Source: CAD feature listing. Evaluate the final solid. Frame: model axes, mm. A direction names the side the tool comes from. Give positions to 0.01 mm unless a question says otherwise; leave off trailing zeros. Loops run counter-clockwise (first coordinate to the right, second up) from the corner with the lowest first, then second, coordinate; pieces in that order, holes last.
```python
from build123d import *

# Parameters (mm, degrees)
EXTRUDE_1_DEPTH     = 1.5
SKETCH_3_R          = 0.9
EXTRUDE_2_DEPTH     = 2
SKETCH_4_R          = 0.9
EXTRUDE_3_DEPTH     = 2
SKETCH_5_R          = 1.1
EXTRUDE_4_DEPTH     = 2
FILLET_1_R          = 2
SKETCH_6_R          = 0.9
CUT_EXTRUDE_1_DEPTH = 10
SKETCH_7_R          = 1
CUT_EXTRUDE_2_DEPTH = 10
SKETCH_8_R          = 0.9
EXTRUDE_5_DEPTH     = 3
CUT_EXTRUDE_3_DEPTH = 3


with BuildPart() as part:
    # 草图1 → 凸台-拉伸1 (new body)
    with BuildSketch(Plane(origin=(0, 0, 0), x_dir=(1, 0, 0), z_dir=(0, 1, 0))):
        Polygon((15.5, 26.846787517), (-15.5, 26.846787517), (-31, 0), (-15.5, -26.846787517), (15.5, -26.846787517), (31, 0), align=None)
    extrude(amount=EXTRUDE_1_DEPTH)

    # 草图3 → 凸台-拉伸2 (add)
    with BuildSketch(Plane(origin=(16, 0, 0), x_dir=(0, 0, -1), z_dir=(1, 0, 0))):
        Polygon((-4, 1.5), (-2.5, 8.5), (2.5, 8.5), (4, 1.5), align=None)
        with Locations((0, 6)):
            Circle(SKETCH_3_R, mode=Mode.SUBTRACT)
    extrude_2 = extrude(amount=-EXTRUDE_2_DEPTH)

    # 草图4 → 凸台-拉伸3 (add)
    with BuildSketch(Plane(origin=(17.8, 0, 0), x_dir=(0, 0, -1), z_dir=(1, 0, 0))):
        Polygon((-4, 1.5), (4, 1.5), (2.5, 8.5), (-2.5, 8.5), align=None)
        with Locations((0, 6)):
            Circle(SKETCH_4_R, mode=Mode.SUBTRACT)
    extrude_3 = extrude(amount=EXTRUDE_3_DEPTH)

    # 镜向3: 凸台-拉伸2, 凸台-拉伸3 across plane
    add(extrude_2.mirror(Plane(origin=(0, 0, 0), x_dir=(0, 0, 1), z_dir=(1, 0, 0))))
    add(extrude_3.mirror(Plane(origin=(0, 0, 0), x_dir=(0, 0, 1), z_dir=(1, 0, 0))))

    # 草图5 → 凸台-拉伸4 (add)
    with BuildSketch(Plane(origin=(5, 0, 0), x_dir=(0, 0, -1), z_dir=(1, 0, 0))):
        Polygon((-19.8, 10.5), (-15.5, 10.5), (-15.5, 1.5), (-23.5, 1.5), align=None)
        with Locations((-17.7, 7.9)):
            Circle(SKETCH_5_R, mode=Mode.SUBTRACT)
        Polygon((8.5, 10.5), (8.5, 1.5), (16.5, 1.5), (12.8, 10.5), align=None)
        with Locations(Location((10.7, 7.9, 0), (0, 0, 180))):  # turned: the seam where the file's is
            Circle(SKETCH_5_R, mode=Mode.SUBTRACT)
    extrude(amount=-EXTRUDE_4_DEPTH)

    # 圆角1
    fillet_1_edges = [part.edges().sort_by_distance(p)[0] for p in [
        (31, 0.75, 0),
        (15.5, 0.75, 26.846787517),
        (-15.5, 0.75, 26.846787517),
        (-31, 0.75, 0),
        (-15.5, 0.75, -26.846787517),
        (15.5, 0.75, -26.846787517),
    ]]
    fillet(fillet_1_edges, radius=FILLET_1_R)

    # 草图6 → 切除-拉伸1 (cut)
    with BuildSketch(Plane.XZ):
        with Locations(Location((-14, 24.25, 0), (0, 0, 270))):  # turned: the seam where the file's is
            Circle(SKETCH_6_R)
        with Locations(Location((14, 24.25, 0), (0, 0, 90))):  # turned: the seam where the file's is
            Circle(SKETCH_6_R)
        with Locations(Location((14, -24.25, 0), (0, 0, 270))):  # turned: the seam where the file's is
            Circle(SKETCH_6_R)
        with Locations(Location((-14, -24.25, 0), (0, 0, 90))):  # turned: the seam where the file's is
            Circle(SKETCH_6_R)
        with BuildLine():
            Line((-14.97853003, 19.25), (-12.344555434, 19.25))
            ThreePointArc((-12.344555434, 19.25), (-11.283895262, 18.810660172), (-10.844555434, 17.75))
            Line((-10.844555434, 17.75), (-10.844555434, 10.75))
            ThreePointArc((-10.844555434, 10.75), (-11.283895262, 9.689339828), (-12.344555434, 9.25))
            Line((-12.344555434, 9.25), (-19.019981914, 9.25))
            ThreePointArc((-19.019981914, 9.25), (-20.31902002, 10), (-20.31902002, 11.5))
            Line((-20.31902002, 11.5), (-16.277568136, 18.5))
            ThreePointArc((-16.277568136, 18.5), (-15.72853003, 19.049038106), (-14.97853003, 19.25))
        make_face()
    extrude(amount=-CUT_EXTRUDE_1_DEPTH, mode=Mode.SUBTRACT)

    # 草图7 → 切除-拉伸2 (cut)
    with BuildSketch(Plane.XZ):
        with Locations(Location((-7.5, -21.846787517, 0), (0, 0, 270))):  # turned: the seam where the file's is
            Circle(SKETCH_7_R)
        with Locations(Location((7.5, -21.846787517, 0), (0, 0, 90))):  # turned: the seam where the file's is
            Circle(SKETCH_7_R)
        with Locations(Location((7.5, 21.846787517, 0), (0, 0, 270))):  # turned: the seam where the file's is
            Circle(SKETCH_7_R)
        with Locations(Location((-7.5, 21.846787517, 0), (0, 0, 90))):  # turned: the seam where the file's is
            Circle(SKETCH_7_R)
    extrude(amount=-CUT_EXTRUDE_2_DEPTH, mode=Mode.SUBTRACT)

    # 草图8 → 凸台-拉伸5 (add)
    with BuildSketch(Plane.ZY.offset(-14)):
        Polygon((-4, 1.5), (4, 1.5), (2.5, 8.5), (-2.5, 8.5), align=None)
        with Locations(Location((0, 6, 0), (0, 0, 180))):  # turned: the seam where the file's is
            Circle(SKETCH_8_R, mode=Mode.SUBTRACT)
    extrude(amount=EXTRUDE_5_DEPTH)

    # 草图9 → 切除-拉伸3 (cut)
    with BuildSketch(Plane(origin=(19.8, 0, 0), x_dir=(0, 0, -1), z_dir=(1, 0, 0))):
        Polygon((-2.5, 8.5), (-4, 1.5), (4, 1.5), (2.5, 8.5), align=None)
    extrude(amount=-CUT_EXTRUDE_3_DEPTH, mode=Mode.SUBTRACT)


solid = part.part
```
(1) Mould query, pull axis Y, two halves, no side actions, for faces 1 (the cylindrical face through (-15.01, 6.89, 0.12)), 2 (the flat face through (-10.845, 1, 14)), 3 (the flat face through (-19, 8.5, 0)). Classes: pulls with the +Y half, pulls with the -Y half, needs draft (parallel to the pull), parting line crosses it, or undercut.
A:
face 1: undercut
face 2: needs draft
face 3: pulls with the +Y half
(2) Section B-B, the plane x = -7.5. Return the cut outline in (y, z).
A:
outline: (0, -26.85) - (1.5, -26.85) - (1.5, -22.85) - (0, -22.85) - close; (0, -20.85) - (1.5, -20.85) - (1.5, 20.85) - (0, 20.85) - close; (0, 22.85) - (1.5, 22.85) - (1.5, 26.85) - (0, 26.85) - close
(3) Reachability of faces 4 (the cylindrical face through (-11.272, 0.74, 9.701)), 5 (the flat face through (5, 5, 19)), 6 (the flat face through (13.54, 4.95, 3.26)), 7 (the flat face through (-17.8, 4, 0)), 8 (the flat face through (-23.15, 0.74, -13.6)) from +Z, -Z, +X, -X, +Y, -Y: full face, straight path, thin tool, end or side. Return the list, or none.
A:
face 4: +Y, -Y
face 5: +Z, -Z, +X, +Y
face 6: +Z, +X, -X, +Y
face 7: +Z, -Z, +Y
face 8: -Z, -X, +Y, -Y
(4) Section A-A, the plane z = 24.25. Return the cut outline in (x, y).
A:
outline: (-17, 0) - (-14.9, 0) - (-14.9, 1.5) - (-17, 1.5) - close; (-13.1, 0) - (13.1, 0) - (13.1, 1.5) - (-13.1, 1.5) - close; (14.9, 0) - (17, 0) - (17, 1.5) - (14.9, 1.5) - close
(5) Section C-C, the plane y = 9.75. Return the cut outline in (x, z), then the cut area to 3 significant figures.
A:
outline: (3, -13.11) - (5, -13.11) - (5, -8.5) - (3, -8.5) - close; (3, 15.5) - (5, 15.5) - (5, 20.11) - (3, 20.11) - close
area: 18.4 mm2
(6) Section D-D, the plane z = 14.5. Return the cut outline in (x, y), then the cut area to 3 significant figures.
A:
outline: (-22.63, 0) - (-18.59, 0) - (-18.59, 1.5) - (-22.63, 1.5) - close; (-10.84, 0) - (22.63, 0) - (22.63, 1.5) - (-10.84, 1.5) - close
area: 56.3 mm2
(7) First-contact query: pin 1 (1.6 mm diameter, centred on x = -17, y = 1, fed in from +Z); pin 2 (2 mm diameter, centred on x = 4.5, y = 5.5, fed in from +Z); pin 3 (2.5 mm diameter, centred on x = 13, z = 0.5, fed in from +Y); pin 4 (1.6 mm diameter, centred on x = 7.5, z = 21.85, fed in from -Y). Flat tips, straight axial feed; report the tip coordinate or a pass-through.
A:
pin 1: stops at z = 25.63
pin 2: stops at z = 22.27
pin 3: stops at y = 8.5
pin 4: passes through
(8) Ray query, line 1 along X through (y, z) = (3.5, -3); line 2 along Y through (x, z) = (-2, -8.5); line 3 along Z through (x, y) = (14.5, 5.75). Return the intervals inside material, ascending.
A:
line 1: x = -19.8 to -17.8, -16 to -14, 11 to 16
line 2: y = 0 to 1.5
line 3: z = -3.09 to -0.86, 0.86 to 3.09
